from build123d import *

# Parameters (mm, degrees)
REVOLVE1_ANGLE = 180
SKETCH3_W      = 2
SKETCH3_H      = 15


with BuildPart() as part:
    # Sketch1 → Revolve1 (revolve)
    with BuildSketch(Plane.XY):
        Polygon((-19.882341212, 25), (-19.882341212, 11.5), (30.117658788, 11.5), (30.117658788, 25), (23.367658788, 25), (23.367658788, 19), (16.117658788, 19), (14.512644781, 15), (-4.277327206, 15), (-5.882341212, 19), (-13.132341212, 19), (-13.132341212, 25), align=None)
    revolve(axis=Axis((-47.288030425, 0, 0), (1, 0, 0)), revolution_arc=REVOLVE1_ANGLE)

    # Sketch3 → Cut-Revolve1 (revolve, cut)
    with BuildSketch(Plane(origin=(0, 0, 0), x_dir=(1, 0, 0), z_dir=(0, 1, 0))):
        with Locations((4.117658788, -7.5)):
            Rectangle(SKETCH3_W, SKETCH3_H)
    revolve(axis=Axis((5.117658788, 0, 0), (0, 0, 1)), mode=Mode.SUBTRACT)


solid = part.part
Source: CAD feature listing. Evaluate the final solid. Frame: model axes, mm. A direction names the side the tool comes from. Round coordinates to 2 decimals unless told otherwise and drop trailing zeros. Write each loop counter-clockwise with the first axis right and the second up, starting at its lowest first coordinate (ties: lowest second). Pieces come first, ordered by that corner, then holes. Notation, with made-up numbers: M 19.5,28.25 L 29.5,28.25 A21 ccw 29.5,55.25 Z; hole C 29,-7.5 d8. An arc over 180 degrees is marked long. One line per item, written item: value. Start each with the question number.
Item 1: Section query C-C (x = -15.5). Return the cut outline in (y, z).
Item 2: Section query B-B (x = 20). Return the cut outline in (y, z), plus the area to 3 significant figures.
Item 3: Ray query, L1, parallel to X at y = 0, z = 14.1; L2, parallel to X at y = 0, z = 21.75; L3, parallel to Y at x = 16.5, z = 9.75. Return the intervals inside material, ascending. Write a range as from..to.
Item 4: Section query A-A (y = 0). Return the cut outline in (x, z).
Item 5: Set-up query: faces 1 (the conical face through (14.59, 0.33, 15.19)), 2 (the cylindrical face through (5.468, 4.17, 10.717)). Return all of +Z, -Z, +X, -X, +Y, -Y with unobstructed straight access to the full face (end or side cutting, diameter ignored); none if empty.
Item 6: Pin query (flat end, axial travel): pin 1 (1.5 mm diameter, centred on x = 16, y = -5.5, fed in from +Z); pin 2 (3 mm diameter, centred on x = -12.5, y = -18, fed in from +Z); pin 3 (4 mm diameter, centred on x = 22.5, z = 13, fed in from +Y). Return the tip coordinate at first contact, or that it passes through.
Result set:
1. outline: M -25,0 L -11.5,0 A11.5 cw 11.5,0 L 25,0 A25 ccw Z
2. outline: M -19,0 L -11.5,0 A11.5 cw 11.5,0 L 19,0 A19 ccw Z
2. area: 359 mm²
3. L1: x = -19.88..3.12, 7.12..30.12
3. L2: x = -19.88..-13.13, 23.37..30.12
3. L3: y = -16.31..-6.1, 6.1..16.31
4. outline: M -19.88,11.5 L 3.12,11.5 L 3.12,15 L -4.28,15 L -5.88,19 L -13.13,19 L -13.13,25 L -19.88,25 Z; M 7.12,11.5 L 30.12,11.5 L 30.12,25 L 23.37,25 L 23.37,19 L 16.12,19 L 14.51,15 L 7.12,15 Z
5. face 1: +Z
5. face 2: -Z, +X, -X
6. pin 1: stops at z = 18.39
6. pin 2: stops at z = 18.66
6. pin 3: stops at y = 22.35
